```python
from build123d import *

# Parameters (mm, degrees)
F0_W     = 228.6
F0_H     = 939.8
F1_DEPTH = 8.1788
F2_W     = 3.175
F2_H     = 3.175
F3_DEPTH = 939.801


with BuildPart() as f1:
    # F0 (on Front) → F1 (new body)
    with BuildSketch(Plane.XZ):
        Rectangle(F0_W, F0_H)
    extrude(amount=F1_DEPTH)

    # F2 (on face) → F3 (cut, through all)
    with BuildSketch(Plane.XY.offset(469.9)):
        with Locations((-87.3125, -6.5913)):
            Rectangle(F2_W, F2_H)
        with Locations((-80.9625, -6.5913)):
            Rectangle(F2_W, F2_H)
        with Locations((-36.5125, -6.5913)):
            Rectangle(F2_W, F2_H)
        with Locations((-30.1625, -6.5913)):
            Rectangle(F2_W, F2_H)
        with Locations((14.2875, -6.5913)):
            Rectangle(F2_W, F2_H)
        with Locations((20.6375, -6.5913)):
            Rectangle(F2_W, F2_H)
        with Locations((65.0875, -6.5913)):
            Rectangle(F2_W, F2_H)
        with Locations((71.4375, -6.5913)):
            Rectangle(F2_W, F2_H)
    extrude(amount=-F3_DEPTH, mode=Mode.SUBTRACT)


solid = f1.part
```
Build history of the part. All positions in model axes, mm. Coordinates: 2 decimals unless noted, no trailing zeros.
1. Drop a flat-ended pin along its axis: pin 1 (2.5 mm diameter, centred on x = 14, z = -44, fed in from -Y). Give the stop position or say it passes through.
Answer block:
pin 1: stops at y = -5
2. Band-saw the part on A-A, the plane y = -6.5. Give the number of separate pieces and of enclosed holes in the cut face, and give its area (3 significant figures).
Answer block:
separate pieces: 9
enclosed holes: 0
area: 191,000 mm2
3. Drill centre line: probe 1 along Y at (x, z) = (-82.5, -409.5). Where is it in solid material? Low to high.
Answer block:
probe 1: y = -5 to 0
